from build123d import *

# Parameters (mm, degrees)
F1_DEPTH = 150
F3_D     = 8.5
F3_DEPTH = 16.5
F3_TIP   = 2.5536576309
F5_D     = 10
F5_DEPTH = 25
F5_TIP   = 3.0043030951
F7_D     = 6
F7_DEPTH = 25
F7_TIP   = 1.8025818571
F8_R     = 12


with BuildPart() as f1:
    # F0 (on Top) → F1 (new body)
    with BuildSketch(Plane.XY):
        Polygon((32, -3.5), (32, 0), (0, 0), (0, -32), (3.5, -32), (3.5, -3.5), align=None)
    extrude(amount=F1_DEPTH)

    # F3
    with Locations(Plane.YZ.offset(3.5)):
        with Locations((-17.75, 134), (-17.75, 16)):
            Hole(F3_D / 2, depth=F3_DEPTH)
            with Locations((0, 0, -(F3_DEPTH + F3_TIP / 2))):  # 118° drill point
                Cone(0, F3_D / 2, F3_TIP, mode=Mode.SUBTRACT)

    # F5
    with Locations(Plane.XZ.offset(3.5)):
        with Locations((17.75, 118), (17.75, 32)):
            Hole(F5_D / 2, depth=F5_DEPTH)
            with Locations((0, 0, -(F5_DEPTH + F5_TIP / 2))):  # 118° drill point
                Cone(0, F5_D / 2, F5_TIP, mode=Mode.SUBTRACT)

    # F7
    with Locations(Plane.XZ.offset(3.5)):
        with Locations((17.75, 75)):
            Hole(F7_D / 2, depth=F7_DEPTH)
            with Locations((0, 0, -(F7_DEPTH + F7_TIP / 2))):  # 118° drill point
                Cone(0, F7_D / 2, F7_TIP, mode=Mode.SUBTRACT)

    # F8
    f8_edges = [f1.edges().sort_by_distance(p)[0] for p in [
        (1.75, -32, 150),
        (32, -1.75, 150),
        (32, -1.75, 0),
        (1.75, -32, 0),
    ]]
    fillet(f8_edges, radius=F8_R)


solid = f1.part
Read the model definition and answer for the solid it produces. Units are mm, in the model's axes. A direction names the side the tool comes from. Round coordinates to 2 decimals unless told otherwise and drop trailing zeros. Write each loop counter-clockwise with the first axis right and the second up, starting at its lowest first coordinate (ties: lowest second). Pieces come first, ordered by that corner, then holes.
Q1. Find section C-C on x = 17.75. Determine the outline of the cut face in (y, z).
Values:
outline: (-3.5, 0) - (0, 0) - (0, 27) - (-3.5, 27) - close; (-3.5, 37) - (0, 37) - (0, 72) - (-3.5, 72) - close; (-3.5, 78) - (0, 78) - (0, 113) - (-3.5, 113) - close; (-3.5, 123) - (0, 123) - (0, 150) - (-3.5, 150) - close
Q2. The mould has two halves that part along Z. Classify faces 1 (the face through (28.58, -1.73, 146.39)), 2 (the face through (18.83, -1.73, 113.12)), 3 (the face through (2, -32, 74)), 4 (the face through (28.58, -1.73, 3.61)): released by +Z, released by -Z, zero draft, split by the parting line, or undercut.
Values:
face 1: released by +Z
face 2: undercut
face 3: zero draft
face 4: released by -Z
Q3. Find section D-D on z = 75. Determine the outline of the cut face in (x, y).
Values:
outline: (0, -32) - (3.5, -32) - (3.5, -3.5) - (14.75, -3.5) - (14.75, 0) - (0, 0) - close; (20.75, -3.5) - (32, -3.5) - (32, 0) - (20.75, 0) - close
Q4. Flat-ended cylindrical pins translate along their axes: P1, Ø9, axis at x = 17.75, z = 32, coming from the +Y side; P2, Ø14, axis at y = -13.5, z = 107, coming from the +X side; P3, Ø8, axis at x = 22.5, z = 46.5, coming from the -Y side. Find the tip coordinate at first contact, or state that the pin passes through.
Values:
P1: passes through
P2: stops at x = 3.5
P3: stops at y = -3.5
Q5. Find section B-B on z = 32. Determine the outline of the cut face in (x, y), and give its area (3 significant figures).
Values:
outline: (0, -32) - (3.5, -32) - (3.5, -3.5) - (12.75, -3.5) - (12.75, 0) - (0, 0) - close; (22.75, -3.5) - (32, -3.5) - (32, 0) - (22.75, 0) - close
area: 177 mm2
Q6. Straight lines are drawn through the part: line 1 (Z direction, x = 17.75, y = -0.75); line 2 (Z direction, x = 17, y = -2); line 3 (Z direction, x = 22, y = -3). For each, find the intervals that lie inside material, in ascending order.
Values:
line 1: z = 0 to 27, 37 to 72, 78 to 113, 123 to 150
line 2: z = 0 to 27.06, 36.94 to 72.1, 77.9 to 113.06, 122.94 to 150
line 3: z = 0.17 to 29.37, 34.63 to 115.37, 120.63 to 149.83
Q7. A tool of negligible diameter and unlimited length cuts with its end or side. For faces 5 (the face through (32, -2, 74)), 6 (the face through (14, -3.5, 74)), from which of +Z, -Z, +X, -X, +Y, -Y can it reach the whole face along a straight path? Write none if from no direction.
Values:
face 5: +Z, -Z, +X, +Y, -Y
face 6: +Z, -Z, +X, -Y
Q8. Find section A-A on y = -17.75. Determine the outline of the cut face in (x, z), and give its area (4 significant figures).
Values:
outline: (0, 0) - (3.5, 0) - (3.5, 11.75) - (0, 11.75) - close; (0, 20.25) - (3.5, 20.25) - (3.5, 129.75) - (0, 129.75) - close; (0, 138.25) - (3.5, 138.25) - (3.5, 150) - (0, 150) - close
area: 465.5 mm2
